Design review of the part built by this model. Coordinates are the model's own, in mm. Face numbers are marked on the shaded views. Coordinates: 2 decimals unless noted, no trailing zeros. Write each loop counter-clockwise with the first axis right and the second up, starting at its lowest first coordinate (ties: lowest second). Pieces come first, ordered by that corner, then holes.
Q1. Add section C-C, the plane y = -0.45. Give the boundary of the cut face in (x, z).
Q2. Add section A-A, the plane z = -11.2. Give the boundary of the cut face in (x, y).
Q3. Add section B-B, the plane x = 23.9. Give the boundary of the cut face in (y, z).
Q4. Clearance check with flat-ended pins moving along their axes: pin 1 Ø1.5 at (y, z) = (-1, -11.5) entering from +X; pin 2 Ø1.5 at (y, z) = (-2.5, 7) entering from +X; pin 3 Ø0.9 at (x, y) = (24.5, -1) entering from -Z; pin 4 Ø0.9 at (x, y) = (23.5, -2) entering from +Z. State where each tip first meets the part, or that it passes through.
Q5. The part is to be moulded in two halves that separate along X. For the marked faces 1, 2 and 3, say which applies: +X half, -X half, draft (parallel to the pull), parting line (faces both ways), or undercut.
Q6. Add section D-D, the plane x = 0. Give the boundary of the cut face in (y, z), plus the area to 3 significant figures.
Q7. To check wall thickness, follow probe 1 along X at (y, z) = (-2.2, -11.2); probe 2 along Z at (x, y) = (23.9, -2); probe 3 along X at (y, z) = (-0.9, 0). State the ranges of each line that lie inside material, in increasing order.
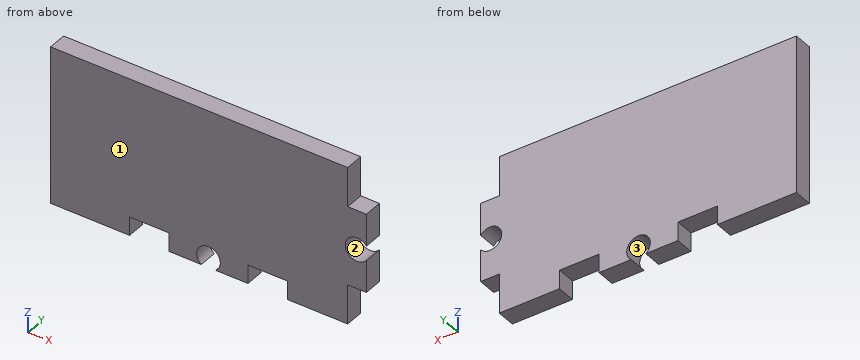
from build123d import *

# Parameters (mm, degrees)
F1_DEPTH = 3
F3_D     = 3.7973
F4_D     = 3.7973


with BuildPart() as f1:
    # F0 (on Front) → F1 (new body)
    with BuildSketch(Plane.XZ):
        Polygon((22.4, 12.7), (-25.4, 12.7), (-25.4, -12.7), (-12.7, -12.7), (-12.7, -9.7), (-6.35, -9.7), (-6.35, -12.7), (6.3499999233, -12.7), (6.3499999233, -9.7), (12.6999999233, -9.7), (12.6999999233, -12.7), (22.4, -12.7), (22.4, -6.35), (25.4, -6.35), (25.4, 6.35), (22.4, 6.35), align=None)
    extrude(amount=F1_DEPTH)

    # F3 (through all)
    with Locations(Plane.XZ.offset(3)):
        with Locations((0, -11.2)):
            Hole(F3_D / 2)

    # F4 (through all)
    with Locations(Plane.XZ.offset(3)):
        with Locations((23.9, 0)):
            Hole(F4_D / 2)


solid = f1.part
Here are the results:
1. outline: (-25.4, -12.7) - (-12.7, -12.7) - (-12.7, -9.7) - (-6.35, -9.7) - (-6.35, -12.7) - (-1.16, -12.7) arc R1.9 cw (long way) to (1.16, -12.7) - (6.35, -12.7) - (6.35, -9.7) - (12.7, -9.7) - (12.7, -12.7) - (22.4, -12.7) - (22.4, -6.35) - (25.4, -6.35) - (25.4, -1.16) arc R1.9 cw (long way) to (25.4, 1.16) - (25.4, 6.35) - (22.4, 6.35) - (22.4, 12.7) - (-25.4, 12.7) - close
2. outline: (-25.4, -3) - (-12.7, -3) - (-12.7, 0) - (-25.4, 0) - close; (-6.35, -3) - (-1.9, -3) - (-1.9, 0) - (-6.35, 0) - close; (1.9, -3) - (6.35, -3) - (6.35, 0) - (1.9, 0) - close; (12.7, -3) - (22.4, -3) - (22.4, 0) - (12.7, 0) - close
3. outline: (-3, -6.35) - (0, -6.35) - (0, -1.9) - (-3, -1.9) - close; (-3, 1.9) - (0, 1.9) - (0, 6.35) - (-3, 6.35) - close
4. pin 1: stops at x = 22.4
4. pin 2: stops at x = 25.4
4. pin 3: stops at z = -6.35
4. pin 4: stops at z = 6.35
5. face 1: draft
5. face 2: undercut
5. face 3: undercut
6. outline: (-3, -9.3) - (0, -9.3) - (0, 12.7) - (-3, 12.7) - close
6. area: 66.0 mm2
7. probe 1: x = -25.4 to -12.7, -6.35 to -1.9, 1.9 to 6.35, 12.7 to 22.4
7. probe 2: z = -6.35 to -1.9, 1.9 to 6.35
7. probe 3: x = -25.4 to 22
